from build123d import *

# Parameters (mm, degrees)
EXTRUDE_1_DEPTH     = 4
EXTRUDE_2_DEPTH     = 4
SKETCH_4_R          = 1.35
SKETCH_4_R_2        = 13
CUT_EXTRUDE_1_DEPTH = 4
SKETCH_5_R          = 1.35
CUT_EXTRUDE_2_DEPTH = 4
EXTRUDE_3_REACH     = 124.967
FILLET_1_R          = 1
CUT_EXTRUDE_3_DEPTH = 4
FILLET_2_R          = 2


with BuildPart() as part:
    # 草图1 → 凸台-拉伸1 (new body)
    with BuildSketch(Plane(origin=(0, 0, 0), x_dir=(1, 0, 0), z_dir=(0, 1, 0))):
        with BuildLine():
            Line((-1.199773028, 28.474735199), (35, 30))
            Line((35, 30), (35, -30))
            Line((35, -30), (-1.199773028, -28.474735199))
            ThreePointArc((-1.199773028, -28.474735199), (-28.5, 0), (-1.199773028, 28.474735199))
        make_face()
    extrude(amount=EXTRUDE_1_DEPTH)

    # 草图3 → 凸台-拉伸2 (add)
    with BuildSketch(Plane(origin=(35, 0, 0), x_dir=(0, 0, -1), z_dir=(1, 0, 0))):
        with BuildLine():
            Line((-30, 0), (-30, 70))
            ThreePointArc((-30, 70), (0, 100), (30, 70))
            Line((30, 70), (30, 0))
            Line((30, 0), (-30, 0))
        make_face()
    extrude(amount=EXTRUDE_2_DEPTH)

    # 草图4 → 切除-拉伸1 (cut)
    with BuildSketch(Plane.ZY.offset(-35)):
        with Locations((0, 90)):
            Circle(SKETCH_4_R)
        with Locations((17.320508076, 60)):
            Circle(SKETCH_4_R)
        with Locations((-17.320508076, 60)):
            Circle(SKETCH_4_R)
        with Locations((0, 70)):
            Circle(SKETCH_4_R_2)
    extrude(amount=-CUT_EXTRUDE_1_DEPTH, mode=Mode.SUBTRACT)

    # 草图5 → 切除-拉伸2 (cut)
    with BuildSketch(Plane.XZ):
        with Locations(Location((-13.435028843, 13.435028843, 0), (0, 0, 270))):
            Circle(SKETCH_5_R)
        with Locations(Location((13.435028843, 13.435028843, 0), (0, 0, 270))):
            Circle(SKETCH_5_R)
        with Locations(Location((13.435028843, -13.435028843, 0), (0, 0, 270))):
            Circle(SKETCH_5_R)
        with Locations(Location((-13.435028843, -13.435028843, 0), (0, 0, 270))):
            Circle(SKETCH_5_R)
    extrude(amount=-CUT_EXTRUDE_2_DEPTH, mode=Mode.SUBTRACT)

    # 凸台-拉伸3: up to this plane
    extrude_3_end = Plane(origin=(35, 4, 30), z_dir=(0.04209729923272397, 0, -0.9991135157715116))
    # 草图6 → 凸台-拉伸3 (add, up to the surface)
    with BuildSketch(Plane(origin=(0, 0, -30), x_dir=(-1, 0, 0), z_dir=(0, 0, -1)), mode=Mode.PRIVATE) as extrude_3_sk1:
        Polygon((-35, 9), (-35, 4), (-30, 4), align=None)
    extrude_3_tool1 = split(extrude(extrude_3_sk1.sketch, amount=-EXTRUDE_3_REACH, mode=Mode.PRIVATE), bisect_by=extrude_3_end, keep=Keep.BOTH, mode=Mode.PRIVATE)
    add(extrude_3_tool1.solids().sort_by_distance((33.333333, 5.666667, -30))[0])

    # 圆角1
    # the kernel refuses this fillet: 1 mm, written as the material it adds along each edge
    with BuildSketch(Plane(origin=(35, 9, -30), x_dir=(-0.7071067811865455, -0.7071067811865497, 0), z_dir=(0, 0, 1))) as fillet_1_piece_1_section:
        with BuildLine():
            CenterArc((FILLET_1_R * 0.414213562373, -FILLET_1_R), FILLET_1_R, 90, 45)
            Line((-FILLET_1_R * 0.292893218813, -FILLET_1_R * 0.292893218813), (0, 0))
            Line((0, 0), (FILLET_1_R * 0.414213562373, 0))
        make_face()
    fillet_1_piece_1 = extrude(amount=61.035533906, mode=Mode.PRIVATE)
    fillet_1_piece_1 = split(fillet_1_piece_1, bisect_by=Plane(origin=(33.678090618, 9.024924819, 29.94430181), z_dir=(0.042097299232723984, 0, -0.9991135157715116)), keep=Keep.TOP, mode=Mode.PRIVATE)
    add(fillet_1_piece_1)
    with BuildSketch(Plane(origin=(30, 4, -30.824860651), x_dir=(0.7071067811865442, 0.7071067811865507, 0), z_dir=(0, 0, 1))) as fillet_1_piece_2_section:
        with BuildLine():
            CenterArc((FILLET_1_R * 0.414213562373, FILLET_1_R), FILLET_1_R, 225, 45)
            Line((-FILLET_1_R * 0.292893218813, FILLET_1_R * 0.292893218813), (0, 0))
            Line((0, 0), (FILLET_1_R * 0.414213562373, 0))
        make_face()
    fillet_1_piece_2 = extrude(amount=61.649721303, mode=Mode.PRIVATE)
    fillet_1_piece_2 = split(fillet_1_piece_2, bisect_by=Plane(origin=(28.722202674, 4.060172408, -29.735487201), z_dir=(0.042097299232723984, 0, 0.9991135157715116)), keep=Keep.TOP, mode=Mode.PRIVATE)
    fillet_1_piece_2 = split(fillet_1_piece_2, bisect_by=Plane(origin=(28.722202674, 4.060172408, 29.735487201), z_dir=(0.042097299232723984, 0, -0.9991135157715116)), keep=Keep.TOP, mode=Mode.PRIVATE)
    add(fillet_1_piece_2)

    # 草图7 → 切除-拉伸3 (cut)
    with BuildSketch(Plane.ZY.offset(-35)):
        with BuildLine():
            Line((-24, 35), (-16, 35))
            ThreePointArc((-16, 35), (-15.292893219, 34.707106781), (-15, 34))
            Line((-15, 34), (-15, 15.414213562))
            ThreePointArc((-15, 15.414213562), (-15.292893219, 14.707106781), (-16, 14.414213562))
            Line((-16, 14.414213562), (-24, 14.414213562))
            ThreePointArc((-24, 14.414213562), (-24.707106781, 14.707106781), (-25, 15.414213562))
            Line((-25, 15.414213562), (-25, 34))
            ThreePointArc((-25, 34), (-24.707106781, 34.707106781), (-24, 35))
        make_face()
        with BuildLine():
            Line((-11.666666667, 34), (-11.666666667, 15.414213562))
            ThreePointArc((-11.666666667, 15.414213562), (-11.373773448, 14.707106781), (-10.666666667, 14.414213562))
            Line((-10.666666667, 14.414213562), (-2.666666667, 14.414213562))
            ThreePointArc((-2.666666667, 14.414213562), (-1.959559885, 14.707106781), (-1.666666667, 15.414213562))
            Line((-1.666666667, 15.414213562), (-1.666666667, 34))
            ThreePointArc((-1.666666667, 34), (-1.959559885, 34.707106781), (-2.666666667, 35))
            Line((-2.666666667, 35), (-10.666666667, 35))
            ThreePointArc((-10.666666667, 35), (-11.373773448, 34.707106781), (-11.666666667, 34))
        make_face()
        with BuildLine():
            Line((1.666666667, 34), (1.666666667, 15.414213562))
            ThreePointArc((1.666666667, 15.414213562), (1.959559885, 14.707106781), (2.666666667, 14.414213562))
            Line((2.666666667, 14.414213562), (10.666666667, 14.414213562))
            ThreePointArc((10.666666667, 14.414213562), (11.373773448, 14.707106781), (11.666666667, 15.414213562))
            Line((11.666666667, 15.414213562), (11.666666667, 34))
            ThreePointArc((11.666666667, 34), (11.373773448, 34.707106781), (10.666666667, 35))
            Line((10.666666667, 35), (2.666666667, 35))
            ThreePointArc((2.666666667, 35), (1.959559885, 34.707106781), (1.666666667, 34))
        make_face()
        with BuildLine():
            Line((15, 34), (15, 15.414213562))
            ThreePointArc((15, 15.414213562), (15.292893219, 14.707106781), (16, 14.414213562))
            Line((16, 14.414213562), (24, 14.414213562))
            ThreePointArc((24, 14.414213562), (24.707106781, 14.707106781), (25, 15.414213562))
            Line((25, 15.414213562), (25, 34))
            ThreePointArc((25, 34), (24.707106781, 34.707106781), (24, 35))
            Line((24, 35), (16, 35))
            ThreePointArc((16, 35), (15.292893219, 34.707106781), (15, 34))
        make_face()
    extrude(amount=-CUT_EXTRUDE_3_DEPTH, mode=Mode.SUBTRACT)

    # 圆角2
    fillet_2_edges = [part.edges().sort_by_distance(p)[0] for p in [
        (39, 0, 0),
    ]]
    fillet(fillet_2_edges, radius=FILLET_2_R)


solid = part.part
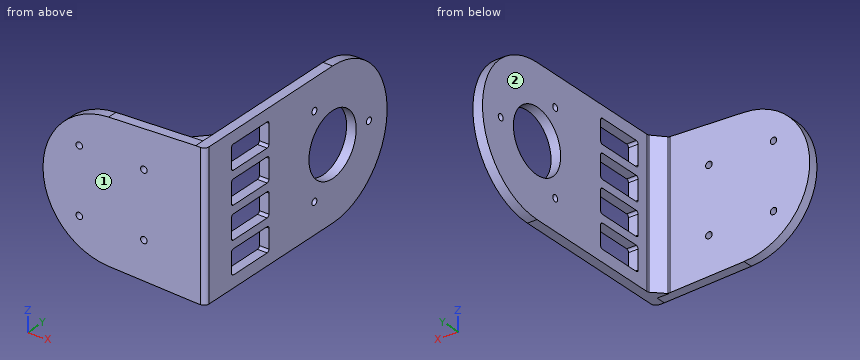
Could you check a few things on this model? Use its own coordinates, in mm. Face numbers are marked on the shaded views. A direction names the side the tool comes from. Give positions to 0.01 mm unless a question says otherwise; leave off trailing zeros. Loops run counter-clockwise (first coordinate to the right, second up) from the corner with the lowest first, then second, coordinate; pieces in that order, holes last. Notation, with made-up numbers: (37.5, 34) -> (92.5, 34) arc R5 ccw to (92.5, 39) -> close; hole circle Ø5 at (3, 35). An arc over 180 degrees is marked (long way). Answer as CSV lines item,"result". Start each with the question number.
(1) Which directions (+Z, -Z, +X, -X, +Y, -Y) give clear straight access to the entire face, cutting with the end or side of a thin tool? Please do the marked faces 1 and 2.
(2) If we section it at D-D on y = 90: Write out the boundary of the cut face in (x, z).
(3) If we section it at A-A on z = 0: Write out the boundary of the cut face in (x, y), then the cut area to 3 significant figures.
(4) If we section it at B-B on z = -20: Write out the boundary of the cut face in (x, y).
(5) I need wall thicknesses on probe 1 along Y at (x, z) = (37, 0); probe 2 along X at (y, z) = (44.5, 16); probe 3 along Y at (x, z) = (-11.5, -3.5). Which ranges of each line are inside material? Lowest first, please.
(6) If we section it at C-C on y = 60: Write out the boundary of the cut face in (x, z), then the cut area to 3 significant figures.
(7) I'm going to push flat-ended pins straight in: pin 1 Ø3 at (x, z) = (31.5, -0.5) entering from +Y; pin 2 Ø1.2 at (x, z) = (37, -22) entering from +Y; pin 3 Ø6 at (y, z) = (41, 16.5) entering from -X. Where does each tip first touch, or does it pass through?
Computed:
1,face 1,"+Z, -Z, +X, -X, -Y"
1,face 2,"+Z, -Z, -X, +Y"
2,outline,"(35, -22.36) -> (39, -22.36) -> (39, -1.35) -> (35, -1.35) -> close; (35, 1.35) -> (39, 1.35) -> (39, 22.36) -> (35, 22.36) -> close"
3,outline,"(-28.5, 0) -> (37, 0) arc R2 ccw to (39, 2) -> (39, 57) -> (35, 57) -> (35, 9.41) arc R1 cw to (34.71, 8.71) -> (30.29, 4.29) arc R1 cw to (29.59, 4) -> (-28.5, 4) -> close; (35, 83) -> (39, 83) -> (39, 88.65) -> (35, 88.65) -> close; (35, 91.35) -> (39, 91.35) -> (39, 100) -> (35, 100) -> close"
3,area,"551 mm2"
4,outline,"(-20.3, 0) -> (37, 0) arc R2 ccw to (39, 2) -> (39, 14.41) -> (35, 14.41) -> (35, 9.41) arc R1 cw to (34.71, 8.71) -> (30.29, 4.29) arc R1 cw to (29.59, 4) -> (-20.3, 4) -> close; (35, 35) -> (39, 35) -> (39, 92.36) -> (35, 92.36) -> close"
5,probe 1,"y = 0 to 57, 83 to 88.65, 91.35 to 100"
5,probe 2,"x = 35 to 39"
5,probe 3,"y = 0 to 4"
6,outline,"(35, -30) -> (39, -30) -> (39, -18.67) -> (35, -18.67) -> close; (35, -15.97) -> (39, -15.97) -> (39, -8.31) -> (35, -8.31) -> close; (35, 8.31) -> (39, 8.31) -> (39, 15.97) -> (35, 15.97) -> close; (35, 18.67) -> (39, 18.67) -> (39, 30) -> (35, 30) -> close"
6,area,"152 mm2"
7,pin 1,"stops at y = 7"
7,pin 2,"stops at y = 91.02"
7,pin 3,"stops at x = 35"
